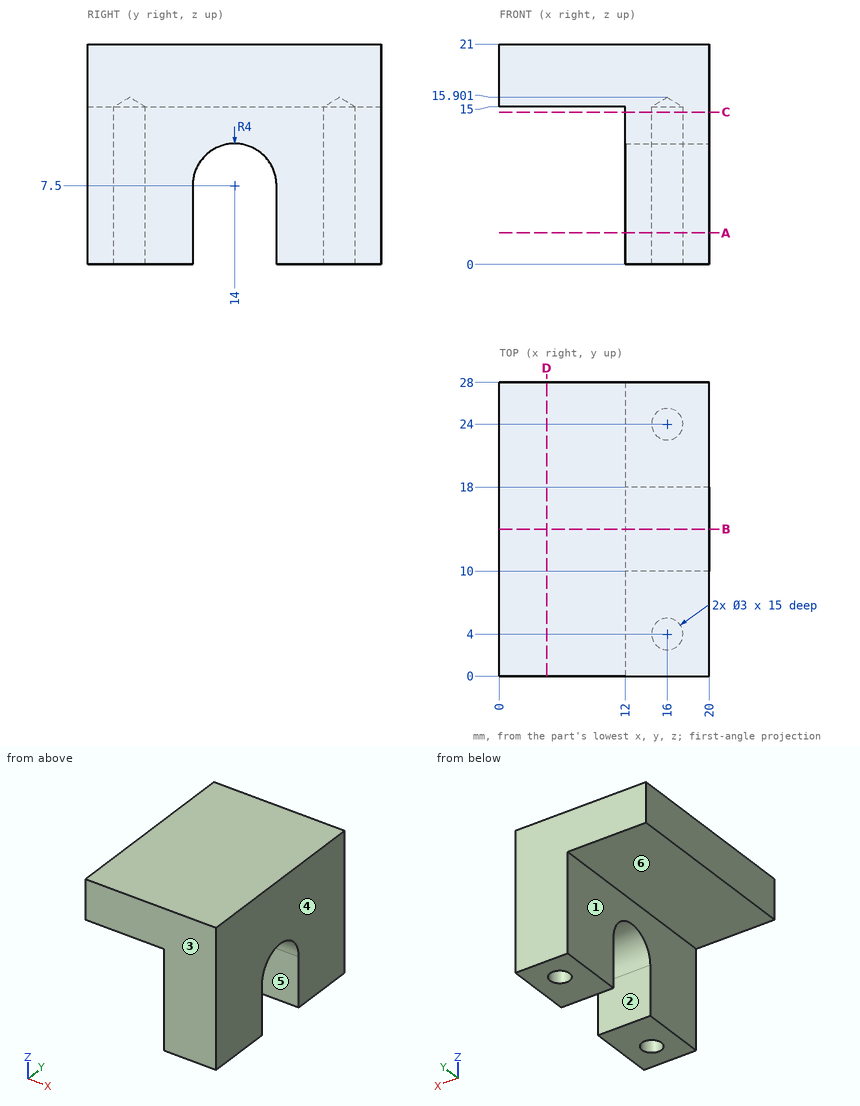
Drawing for the job (mm, zero at the part's lowest x, y, z). A direction names the side the tool comes from. Give positions to 0.01 mm unless a question says otherwise; leave off trailing zeros. Loops run counter-clockwise (first coordinate to the right, second up) from the corner with the lowest first, then second, coordinate; pieces in that order, holes last. Notation, with made-up numbers: M -20.5,44 L 27.5,44 A28 cw 27.5,79 Z; hole C 2,-39 d8. An arc over 180 degrees is marked long. Use one line per item in the form item = value.
Item 1: Slice it at B-B (y = 14). List the corners of the cut face in (x, z).
Determined:
outline = M 0,15 L 12,15 L 12,11.5 L 20,11.5 L 20,21 L 0,21 Z
Item 2: Two-plate mould, pull along Y, no slides. Class the marked faces 1, 2 and 3: pulls with the +Y half, pulls with the -Y half, needs draft (parallel to the pull), parting line crosses it, or undercut.
Determined:
face_1 = needs draft
face_2 = undercut
face_3 = pulls with the -Y half
Item 3: Slice it at C-C (z = 14.5). List the corners of the cut face in (x, y).
Determined:
outline = M 12,0 L 20,0 L 20,28 L 12,28 Z; hole C 16,4 d3; hole C 16,24 d3
Item 4: Which spindle directions (+Z, -Z, +X, -X, +Y, -Y) get a long thin tool onto all of the face, cutting with end or side? Do the marked faces 4, 5 and 6. Say none if no direction does.
Determined:
face_4 = +Z, -Z, +X, +Y, -Y
face_5 = -Z, +X, -X
face_6 = -Z, -X, +Y, -Y
Item 5: Drill centre lines: probe 1 along Y at (x, z) = (16, 7.25); probe 2 along Y at (x, z) = (13.25, 5); probe 3 along X at (y, z) = (4, 7). Where is each one in solid material? Low to high. Write a range as from..to.
Determined:
probe_1 = 0..2.5, 5.5..10, 18..22.5, 25.5..28
probe_2 = 0..10, 18..28
probe_3 = 12..14.5, 17.5..20
Item 6: Flat gauge pins, fed straight in: pin 1 (10 mm diameter, centred on y = 12.5, z = 6, fed in from +X); pin 2 (4.5 mm diameter, centred on y = 11.5, z = 9, fed in from -X); pin 3 (2 mm diameter, centred on x = 5.5, y = 20, fed in from -Z); pin 4 (1.8 mm diameter, centred on x = 16, y = 24, fed in from -Z). Where does each tip first touch, or does it go through?
Determined:
pin_1 = 20
pin_2 = 12
pin_3 = 15
pin_4 = 15.36
Item 7: Slice it at D-D (x = 4.5). List the corners of the cut face in (y, z), plus the area to 3 significant figures.
Determined:
outline = M 0,15 L 28,15 L 28,21 L 0,21 Z
area = 168 mm2
Item 8: Slice it at A-A (z = 3). List the corners of the cut face in (x, y), plus the area to 3 significant figures.
Determined:
outline = M 12,0 L 20,0 L 20,10 L 12,10 Z; M 12,18 L 20,18 L 20,28 L 12,28 Z; hole C 16,4 d3; hole C 16,24 d3
area = 146 mm2
